Job drawing, mm, ordinate dimensions from the low corner. One solid piece. A direction names the side the tool comes from. Coordinates: 2 decimals unless noted, no trailing zeros. Loops run counter-clockwise (first coordinate to the right, second up) from the corner with the lowest first, then second, coordinate; pieces in that order, holes last. Notation, with made-up numbers: M -26.5,17.5 L 9.5,17.5 A27 ccw 9.5,38.5 Z; hole C -29,-11 d9. An arc over 180 degrees is marked long. Answer as a JSON object with one key per item and string values. Group by question number.
1. Saw through at D-D on x = 12.5. Write the cut outline in (y, z).
2. Drop flat-ended pins along their axis: pin 1 Ø1.5 at (y, z) = (9, 5) entering from +X; pin 2 Ø2 at (y, z) = (3.5, 5) entering from -X; pin 3 Ø1 at (y, z) = (8, 6) entering from -X. Give the stop position or say it passes through.
3. 3-axis set-ups, long thin cutter, end or side, ignore diameter. For the marked faces 1 and 2: which of +Z, -Z, +X, -X, +Y, -Y reach the whole face in a straight line?
4. Drill centre lines: L1, parallel to Y at x = 7, z = 0.35; L2, parallel to Y at x = 7, z = 2.4; L3, parallel to X at y = 2.5, z = 0.75. Where is each one in solid material? Low to high.
5. Saw through at C-C on z = 3.5. Write the cut outline in (x, y).
6. Saw through at A-A on y = 7. Write the cut outline in (x, z), then the cut area to 3 significant figures.
7. Mould opens along X. For the marked faces 3, 4 and 5 say: released by +X, released by -X, zero draft, split by the parting line, or undercut.
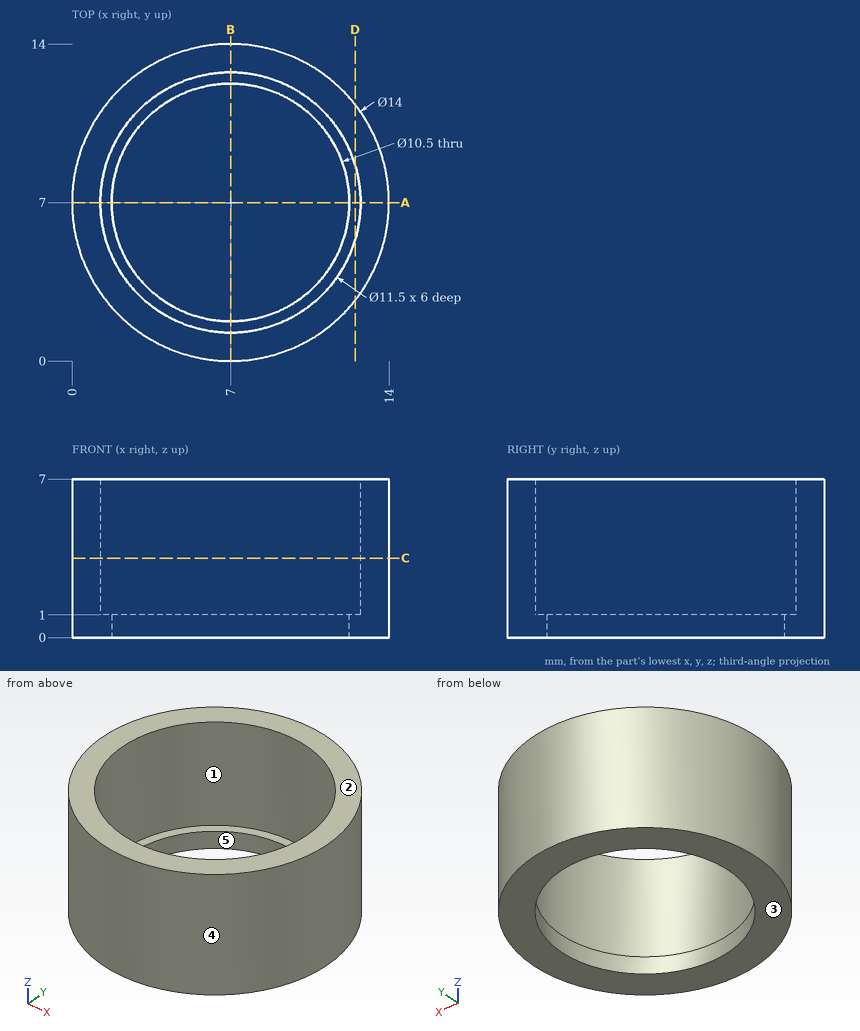
Outcome:
{
 "1": {"outline": "M 2.67,0 L 11.33,0 L 11.33,7 L 8.68,7 L 8.68,1 L 5.32,1 L 5.32,7 L 2.67,7 Z"},
 "2": {"pin 1": "stops at x = 13.89", "pin 2": "stops at x = 0.46", "pin 3": "stops at x = 0.02"},
 "3": {"face 1": "+Z", "face 2": "+Z, +X, -X, +Y, -Y"},
 "4": {"L1": "y = 0 to 1.75, 12.25 to 14", "L2": "y = 0 to 1.25, 12.75 to 14", "L3": "x = 1.64 to 4.3, 9.7 to 12.36"},
 "5": {"outline": "C 7,7 d14; hole C 7,7 d11.5"},
 "6": {"outline": "M 0,0 L 1.75,0 L 1.75,1 L 1.25,1 L 1.25,7 L 0,7 Z; M 12.25,0 L 14,0 L 14,7 L 12.75,7 L 12.75,1 L 12.25,1 Z", "area": "18.5 mm²"},
 "7": {"face 3": "zero draft", "face 4": "split by the parting line", "face 5": "undercut"}
}
